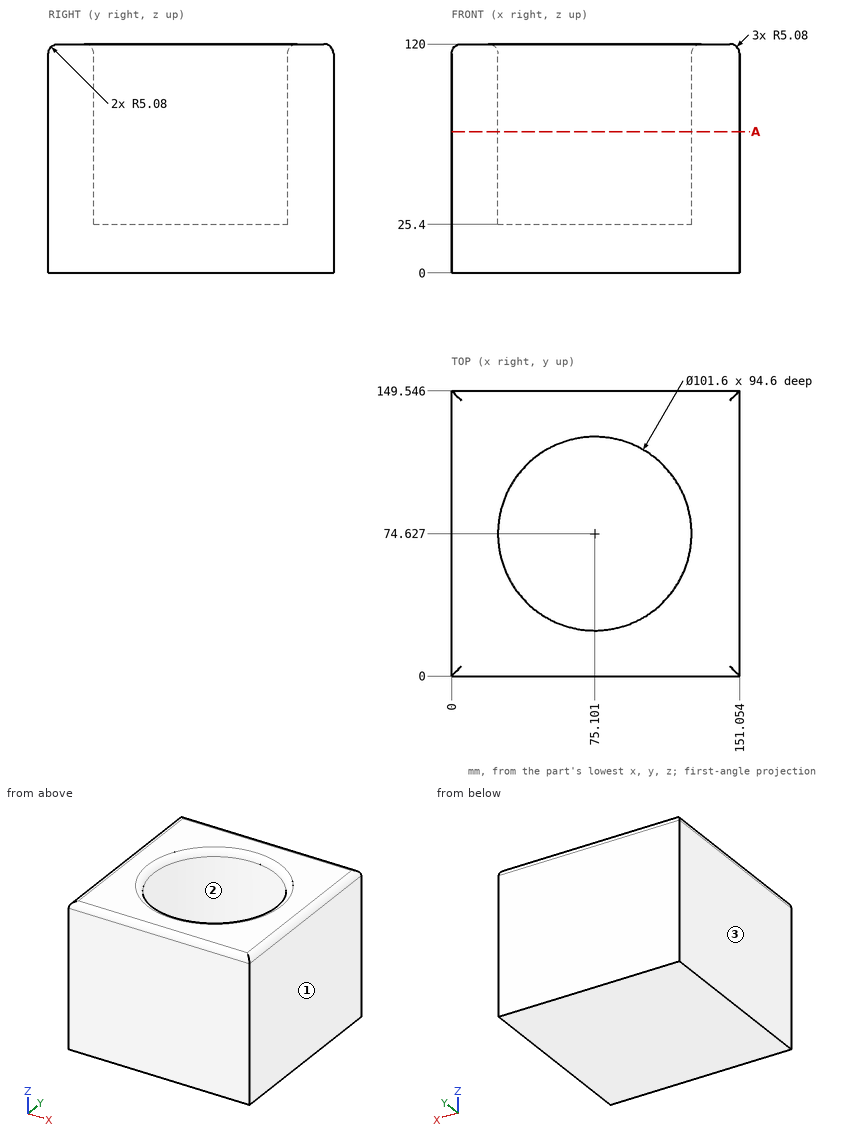
Here's the drawing with two shaded views (mm, measured from the low corner). I have some questions. Coordinates: 2 decimals unless noted, no trailing zeros. Write each loop counter-clockwise with the first axis right and the second up, starting at its lowest first coordinate (ties: lowest second). Pieces come first, ordered by that corner, then holes. Notation, with made-up numbers: M -27,-21 L -12,-21 A20 ccw -12,2 Z; hole C -13.5,58.25 d3. An arc over 180 degrees is marked long. Answer as CSV lines item,"result". Start each with the question number.
1) I want a section at A-A, the plane z = 74. Please give me the cut outline in (x, y).
2) We'd pull the mould along X, two halves only. Please class the marked faces 1, 2 and 3: +X half, -X half, draft (parallel to the pull), parting line (faces both ways), or undercut.
3) Please list where these lines run through material, in increasing order: line 1 (X direction, y = 61.5, z = 65) (1 decimal); line 2 (Z direction, x = 77.5, y = 42.5); line 3 (X direction, y = 107.5, z = 60) (1 decimal). Write a range as from..to.
4) For P1, Ø2, axis at x = 62, y = 112, coming from the +Z side, with a flat end and sliding along its axis, tell me the tip position at first contact or that it passes through.
Data:
1,outline,"M 0,0 L 151.05,0 L 151.05,149.55 L 0,149.55 Z; hole C 75.1,74.63 d101.6"
2,face 1,"+X half"
2,face 2,"undercut"
2,face 3,"-X half"
3,line 1,"x = 0..26, 124.2..151.1"
3,line 2,"z = 0..25.4"
3,line 3,"x = 0..36.4, 113.8..151.1"
4,P1,"stops at z = 25.4"
